Read the model definition and answer for the solid it produces. Units are mm, in the model's axes. Coordinates: 2 decimals unless noted, no trailing zeros. Order: outer loops, then holes, each group sorted by start corner. A loop starts at its lowest first (then second) coordinate and runs counter-clockwise, first axis right, second up.
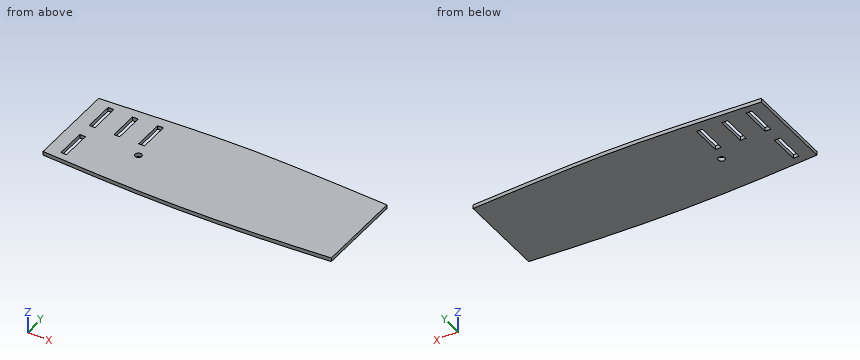
from build123d import *

# Parameters (mm, degrees)
F0_W     = 3
F0_H     = 15.95455
F0_H_2   = 15.564595
F1_DEPTH = 2
F2_R     = 1.709906
F3_DEPTH = 25


with BuildPart() as f1:
    # F0 (on Top) → F1 (new body)
    with BuildSketch(Plane.XY):
        with BuildLine():
            add(Edge.make_bspline(
                [(-75.74358, 23.504223), (-50.49572, 24.757731), (0, 28.379784), (50.49572, 24.757731), (75.74358, 23.504223)],
                knots=[0, 0, 0, 0, 75.805549, 151.611099, 151.611099, 151.611099, 151.611099], degree=3))
            Line((-75.74358, 23.504223), (-75.74358, -23.504223))
            add(Edge.make_bspline(
                [(-75.74358, -23.504223), (-50.49572, -25.16658), (0, -27.970934), (50.49572, -25.16658), (75.74358, -23.504223)],
                knots=[0, 0, 0, 0, 75.805549, 151.611099, 151.611099, 151.611099, 151.611099], degree=3))
            Line((75.74358, -23.504223), (75.74358, 23.504223))
        make_face()
        with Locations((-67.065108, -11.977275)):
            Rectangle(F0_W, F0_H, mode=Mode.SUBTRACT)
        with Locations((-67.065108, 11.977275)):
            Rectangle(F0_W, F0_H, mode=Mode.SUBTRACT)
        with Locations((-54.065108, 11.782298)):
            Rectangle(F0_W, F0_H_2, mode=Mode.SUBTRACT)
        with Locations((-41.065108, 11.977275)):
            Rectangle(F0_W, F0_H, mode=Mode.SUBTRACT)
    extrude(amount=F1_DEPTH)

    # F2 (on face) → F3 (cut)
    with BuildSketch(Plane.XY.offset(2)):
        with Locations((-38.084775, -3.431539)):
            Circle(F2_R)
    extrude(amount=-F3_DEPTH, mode=Mode.SUBTRACT)


solid = f1.part
Q1. Each of these flat-tipped pins is pushed along its axis until it touches: P1, Ø0.6, axis at x = -67, z = 1.5, coming from the +Y side; P2, Ø1, axis at x = -54, z = 1, coming from the -Y side; P3, Ø8, axis at x = -36.5, y = -12.5, coming from the -Z side. Where does it stop, or does it pass through?
Q2. Straight lines are drawn through the part: L1, parallel to X at y = 16.5, z = 1.9; L2, parallel to X at y = -10, z = 0.3; L3, parallel to X at y = -3.5, z = 1.45. For each, find the intervals that lie inside material, in ascending order.
Q3. The part is cut by section C-C, the plane z = 1.5. State how many separate pieces and enclosed holes the cut face has, then the cut area to 3 significant figures.
Q4. The part is cut by section B-B, the plane y = 8. Determine the outline of the cut face in (x, z), then the cut area to 3 significant figures.
Q5. The part is cut by section A-A, the plane y = -9. Determine the outline of the cut face in (x, z), then the cut area to 3 significant figures.
Computed values:
1. P1: stops at y = 23.97
1. P2: stops at y = -24.87
1. P3: stops at z = 0
2. L1: x = -75.74 to -68.57, -65.57 to -55.57, -52.57 to -42.57, -39.57 to 75.74
2. L2: x = -75.74 to -68.57, -65.57 to 75.74
2. L3: x = -75.74 to -39.79, -36.38 to 75.74
3. separate pieces: 1
3. enclosed holes: 5
3. area: 7,500 mm2
4. outline: (-75.74, 0) - (-68.57, 0) - (-68.57, 2) - (-75.74, 2) - close; (-65.57, 0) - (-55.57, 0) - (-55.57, 2) - (-65.57, 2) - close; (-52.57, 0) - (-42.57, 0) - (-42.57, 2) - (-52.57, 2) - close; (-39.57, 0) - (75.74, 0) - (75.74, 2) - (-39.57, 2) - close
4. area: 285 mm2
5. outline: (-75.74, 0) - (-68.57, 0) - (-68.57, 2) - (-75.74, 2) - close; (-65.57, 0) - (75.74, 0) - (75.74, 2) - (-65.57, 2) - close
5. area: 297 mm2
